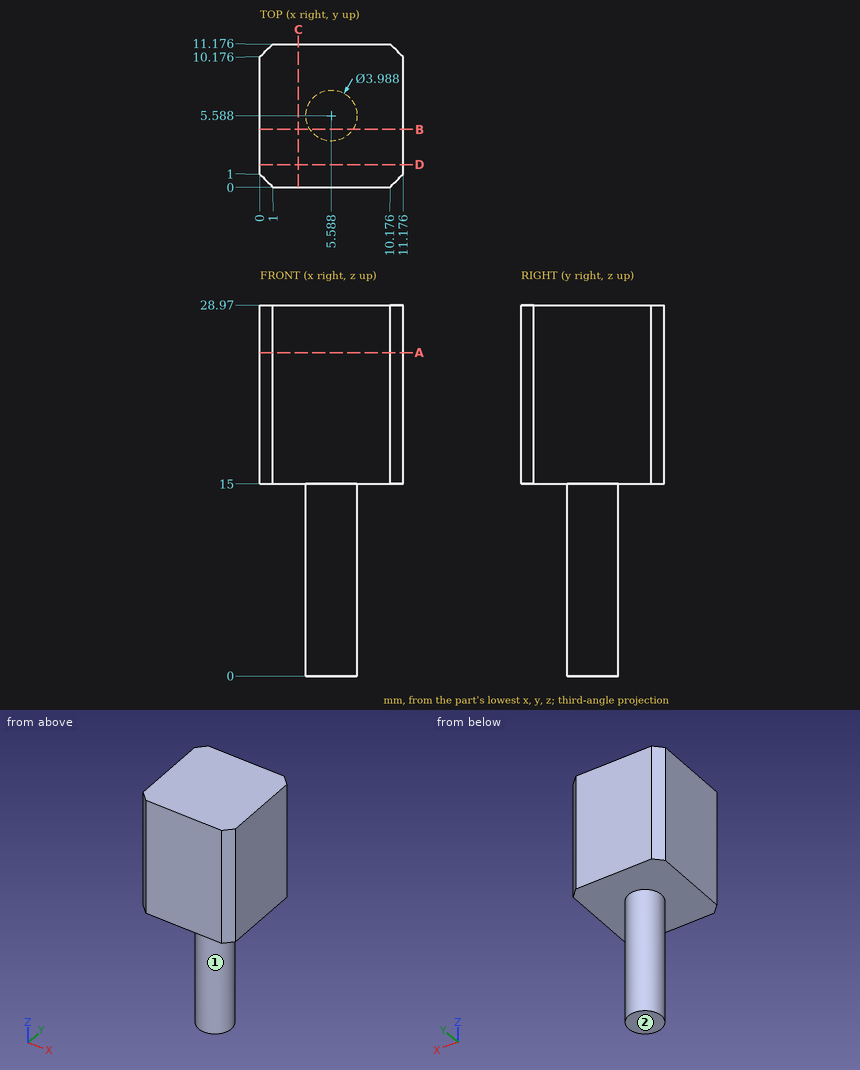
Drawing for the job (mm, zero at the part's lowest x, y, z). A direction names the side the tool comes from. Round coordinates to 2 decimals unless told otherwise and drop trailing zeros. Loops run counter-clockwise (first coordinate to the right, second up) from the corner with the lowest first, then second, coordinate; pieces in that order, holes last.
1. Wall check: probe 1 along Z at (x, y) = (10.25, 4.75); probe 2 along Y at (x, z) = (6.5, 12.75) (1 decimal); probe 3 along X at (y, z) = (6.25, 4.75). Give the ranges that are in metal, low to high.
Check values:
probe 1: z = 15 to 28.97
probe 2: y = 3.8 to 7.4
probe 3: x = 3.71 to 7.47
2. Band-saw the part on A-A, the plane z = 25.25. List the corners of the cut face in (x, y).
Check values:
outline: (0, 1) - (1, 0) - (10.18, 0) - (11.18, 1) - (11.18, 10.18) - (10.18, 11.18) - (1, 11.18) - (0, 10.18) - close
3. Band-saw the part on C-C, the plane x = 3. List the corners of the cut face in (y, z), and give its area (3 significant figures).
Check values:
outline: (0, 15) - (11.18, 15) - (11.18, 28.97) - (0, 28.97) - close
area: 156 mm2
4. Tool access for the marked faces 1 and 2: list every direction of +Z, -Z, +X, -X, +Y, -Y with a clear straight run to the whole face (end or side of a thin tool).
Check values:
face 1: -Z
face 2: -Z, +X, -X, +Y, -Y
5. Drop flat-ended pins along their axis: P1, Ø4, axis at y = 4, z = 5, coming from the -X side; P2, Ø1.5, axis at x = 8.5, y = 9.5, coming from the -Z side. Give the stop position or say it passes through.
Check values:
P1: stops at x = 3.59
P2: stops at z = 15
6. Band-saw the part on B-B, the plane y = 4.5. List the corners of the cut face in (x, z).
Check values:
outline: (0, 15) - (3.92, 15) - (3.92, 0) - (7.26, 0) - (7.26, 15) - (11.18, 15) - (11.18, 28.97) - (0, 28.97) - close
